from build123d import *

# Parameters (mm, degrees)
EXTRUDE_1_DEPTH     = 100
CUT_EXTRUDE_1_REACH = 106.163
SKETCH_2_R          = 5


with BuildPart() as part:
    # Эскиз1 → Бобышка-Вытянуть1 (new body)
    with BuildSketch(Plane.XY):
        with BuildLine():
            Line((10, 14.5), (10, 13.5))
            ThreePointArc((10, 13.5), (9.853553391, 13.146446609), (9.5, 13))
            Line((9.5, 13), (-12.5, 13))
            ThreePointArc((-12.5, 13), (-12.853553391, 12.853553391), (-13, 12.5))
            Line((-13, 12.5), (-13, -9.5))
            ThreePointArc((-13, -9.5), (-13.146446609, -9.853553391), (-13.5, -10))
            Line((-13.5, -10), (-14.5, -10))
            ThreePointArc((-14.5, -10), (-14.853553391, -9.853553391), (-15, -9.5))
            Line((-15, -9.5), (-15, 15))
            Line((-15, 15), (9.5, 15))
            ThreePointArc((9.5, 15), (9.853553391, 14.853553391), (10, 14.5))
        make_face()
    extrude(amount=EXTRUDE_1_DEPTH)

    # Эскиз2 → Вырез-Вытянуть1 (cut, up to next)
    with BuildSketch(Plane(origin=(0, 15, 0), x_dir=(1, 0, 0), z_dir=(0, 1, 0)), mode=Mode.PRIVATE) as cut_extrude_1_sk1:
        with Locations(Location((0, -80, 0), (0, 0, 270))):
            Circle(SKETCH_2_R)
    cut_extrude_1_tool1 = extrude(cut_extrude_1_sk1.sketch, amount=-CUT_EXTRUDE_1_REACH, mode=Mode.PRIVATE) & part.part
    # Эскиз2 → Вырез-Вытянуть1 (cut, up to next)
    with BuildSketch(Plane(origin=(0, 15, 0), x_dir=(1, 0, 0), z_dir=(0, 1, 0)), mode=Mode.PRIVATE) as cut_extrude_1_sk2:
        with Locations(Location((0, -20, 0), (0, 0, 270))):
            Circle(SKETCH_2_R)
    cut_extrude_1_tool2 = extrude(cut_extrude_1_sk2.sketch, amount=-CUT_EXTRUDE_1_REACH, mode=Mode.PRIVATE) & part.part
    add(cut_extrude_1_tool1.solids().sort_by_distance((0, 15, 80))[0], mode=Mode.SUBTRACT)
    add(cut_extrude_1_tool2.solids().sort_by_distance((0, 15, 20))[0], mode=Mode.SUBTRACT)


solid = part.part
For this review, take the finished solid that the model builds, in its own axes (mm). A direction names the side the tool comes from. Give positions to 0.01 mm unless a question says otherwise; leave off trailing zeros. Loops run counter-clockwise (first coordinate to the right, second up) from the corner with the lowest first, then second, coordinate; pieces in that order, holes last.
Item 1: Tool access review of faces 1 (the flat face through (-3, 15, 49)), 2 (the flat face through (-13, 2, 49)): name each direction out of +Z, -Z, +X, -X, +Y, -Y from which nothing blocks a thin tool from reaching the whole face with its end or side.
Item 2: Take a section at D-D, the plane x = 8. State the section outline as (y, z) points.
Item 3: For line 1 along X through (y, z) = (13.7, 20); line 2 along Y through (x, z) = (-11, 6.5); line 3 along X through (y, z) = (9.25, 46), list the stretches that pass through material, from the lowest coordinate up.
Item 4: Take a section at C-C, the plane z = 55. State the section outline as (x, y) points.
Item 5: Draft analysis for pull direction Z (two halves, no side actions). For faces 3 (the cylindrical face through (0, 14, 15)), 4 (the cylindrical face through (-1.915, 14.014, 84.619)), 5 (the flat face through (-8, 14, 100)), 6 (the flat face through (-8, 14, 0)), state which applies: +Z half, -Z half, draft (parallel to the pull), parting line (faces both ways), or undercut.
Item 6: Insertion check: pin 1 (8 mm diameter, centred on x = -10.5, y = 0.5, fed in from +Z); pin 2 (1 mm diameter, centred on y = 3.5, z = 16, fed in from +X); pin 3 (11 mm diameter, centred on x = -2.5, z = 45.5, fed in from -Y). Each pin has a flat end and moves straight along its axis. Give the tip position at first contact, or say it passes through.
Item 7: Take a section at B-B, the plane x = 0. State the section outline as (y, z) points.
Item 8: Take a section at A-A, the plane z = 80. State the section outline as (x, y) points.
Calculated:
1. face 1: +Z, -Z, +X, -X, +Y
1. face 2: +Z, -Z, +X, -Y
2. outline: (13, 0) - (15, 0) - (15, 100) - (13, 100) - close
3. line 1: x = -15 to -5, 5 to 10
3. line 2: y = 13 to 15
3. line 3: x = -15 to -13
4. outline: (-15, -9.5) arc R0.5 ccw to (-14.5, -10) - (-13.5, -10) arc R0.5 ccw to (-13, -9.5) - (-13, 12.5) arc R0.5 cw to (-12.5, 13) - (9.5, 13) arc R0.5 ccw to (10, 13.5) - (10, 14.5) arc R0.5 ccw to (9.5, 15) - (-15, 15) - close
5. face 3: undercut
5. face 4: undercut
5. face 5: +Z half
5. face 6: -Z half
6. pin 1: stops at z = 100
6. pin 2: stops at x = -13
6. pin 3: stops at y = 13
7. outline: (13, 0) - (15, 0) - (15, 15) - (13, 15) - close; (13, 25) - (15, 25) - (15, 75) - (13, 75) - close; (13, 85) - (15, 85) - (15, 100) - (13, 100) - close
8. outline: (-15, -9.5) arc R0.5 ccw to (-14.5, -10) - (-13.5, -10) arc R0.5 ccw to (-13, -9.5) - (-13, 12.5) arc R0.5 cw to (-12.5, 13) - (-5, 13) - (-5, 15) - (-15, 15) - close; (5, 13) - (9.5, 13) arc R0.5 ccw to (10, 13.5) - (10, 14.5) arc R0.5 ccw to (9.5, 15) - (5, 15) - close
